Model file for the job. Use its own axes, mm. Face numbers are marked on the shaded views. A direction names the side the tool comes from. Give positions to 0.01 mm unless a question says otherwise; leave off trailing zeros. Order: outer loops, then holes, each group sorted by start corner. A loop starts at its lowest first (then second) coordinate and runs counter-clockwise, first axis right, second up. Notation, with made-up numbers: (34, 42) -> (71, 42) arc R35 ccw to (71, 81) -> close; hole circle Ø11 at (34.5, 63). An arc over 180 degrees is marked (long way). Answer in a Markdown table with one row per item. Add a question column.
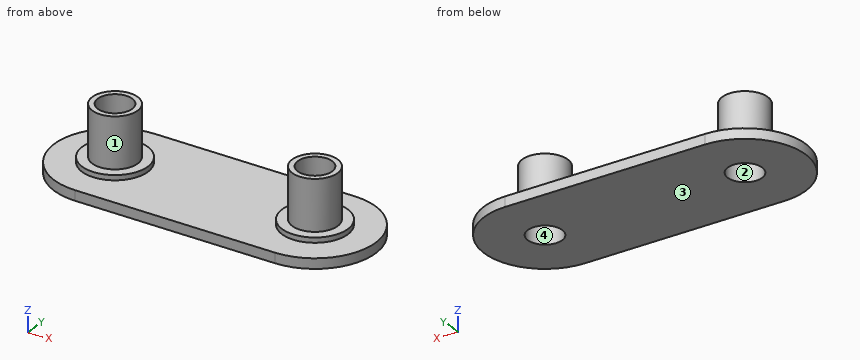
Autodesk Inventor part; units mm, degrees
ref_plane "YZ Plane" through (0, 0, 0) normal (1, 0, 0) x (0, 1, 0)
ref_plane "XZ Plane" through (0, 0, 0) normal (0, 1, 0) x (-1, 0, 0)
ref_plane "XY Plane" through (0, 0, 0) normal (0, 0, 1) x (1, 0, 0)
sketch "Sketch1" plane through (0, 0, 0) normal (0, 0, 1) x (1, 0, 0)
  line L0 (-10, 0) -> (10, 0) construction
  line L1 (-10, -6) -> (10, -6)
  line L2 (10, 6) -> (-10, 6)
  arc A0 (-10, 6) -> (-10, -6) centre (-10, 0) ccw
  arc A1 (10, -6) -> (10, 6) centre (10, 0) ccw
  circle A2 centre (-10, 0) radius 1.7
  circle A3 centre (10, 0) radius 1.7
  point P0 (0, 0)
  point P1 (0, 0)
  dimension "d0" = 20
  dimension "d1" = 6
  dimension "d2" = 3.4
extrude "Extrusion1" add sketch "Sketch1" along normal blind 1
sketch "Sketch2" plane through (0, 0, 1) normal (0, 0, 1) x (1, 0, 0)
  circle A0 centre (10, 0) radius 1.7
  circle A1 centre (10, 0) radius 2.25
  circle A2 centre (-10, 0) radius 1.7
  circle A3 centre (-10, 0) radius 2.25
  point P0 (0, 0)
  dimension "d5" = 4.5
  dimension "d6" = 4.5
extrude "Extrusion2" add sketch "Sketch2" along normal blind 5.5
sketch "Sketch3" plane through (0, 0, 1) normal (0, 0, 1) x (1, 0, 0)
  circle A0 centre (10, 0) radius 2.25
  circle A1 centre (-10, 0) radius 2.25
  circle A2 centre (10, 0) radius 2.25
  arc A3 (10, -6) -> (10, 6) centre (10, 0) ccw
  line L0 (10, 6) -> (-10, 6)
  arc A4 (-10, 6) -> (-10, -6) centre (-10, 0) ccw
  line L1 (-10, -6) -> (10, -6)
  circle A5 centre (10, 0) radius 3.25
  circle A6 centre (-10, 0) radius 3.25
  point P0 (0, 0)
  dimension "d9" = 6.5
extrude "Extrusion3" add sketch "Sketch3" along normal blind 0.5 contours A5 | A6
equation "\"d6\" = d5"
properties part number "Belt Retaining Guide"
Item 1: Saw through at C-C on x = 4.5. List the corners of the cut face in (y, z).
Item 2: Saw through at D-D on y = 4. List the corners of the cut face in (x, z), plus the area to 3 significant figures.
Item 3: Which spindle directions (+Z, -Z, +X, -X, +Y, -Y) get a long thin tool onto all of the face, cutting with end or side? Do the marked faces 1 and 2. Say none if no direction does.
Item 4: Saw through at A-A on y = 0. List the corners of the cut face in (x, z), plus the area to 3 significant figures.
Item 5: Two-plate mould, pull along X, no slides. Class the marked faces 3 and 4: pulls with the +X half, pulls with the -X half, needs draft (parallel to the pull), parting line crosses it, or undercut.
Item 6: Saw through at B-B on z = 5.25. List the corners of the cut face in (x, y).
Item 7: Wall check: line 1 (Y direction, x = 10, z = 3.5); line 2 (X direction, y = -1.5, z = 2.5); line 3 (Z direction, x = 6.5, y = 3). Give the ranges that are in metal, low to high.
Item 8: Pin check, flat tips, straight feed: pin 1 Ø6 at (x, y) = (-2.5, -0.5) entering from +Z; pin 2 Ø4.5 at (x, y) = (10, 0) entering from +Z; pin 3 Ø2 at (y, z) = (1, 5.5) entering from -X. Stop position of each tip, or through.
Evaluation:
| question | item | result |
|---|---|---|
| 1 | outline | (-6, 0) -> (6, 0) -> (6, 1) -> (-6, 1) -> close |
| 2 | outline | (-14.47, 0) -> (14.47, 0) -> (14.47, 1) -> (-14.47, 1) -> close |
| 2 | area | 28.9 mm2 |
| 3 | face 1 | +Z |
| 3 | face 2 | +Z, -Z |
| 4 | outline | (-16, 0) -> (-11.7, 0) -> (-11.7, 6.5) -> (-12.25, 6.5) -> (-12.25, 1.5) -> (-13.25, 1.5) -> (-13.25, 1) -> (-16, 1) -> close; (-8.3, 0) -> (8.3, 0) -> (8.3, 6.5) -> (7.75, 6.5) -> (7.75, 1.5) -> (6.75, 1.5) -> (6.75, 1) -> (-6.75, 1) -> (-6.75, 1.5) -> (-7.75, 1.5) -> (-7.75, 6.5) -> (-8.3, 6.5) -> close; (11.7, 0) -> (16, 0) -> (16, 1) -> (13.25, 1) -> (13.25, 1.5) -> (12.25, 1.5) -> (12.25, 6.5) -> (11.7, 6.5) -> close |
| 4 | area | 39.3 mm2 |
| 5 | face 3 | needs draft |
| 5 | face 4 | undercut |
| 6 | outline | circle Ø4.5 at (-10, 0); circle Ø4.5 at (10, 0); hole circle Ø3.4 at (-10, 0); hole circle Ø3.4 at (10, 0) |
| 7 | line 1 | y = -2.25 to -1.7, 1.7 to 2.25 |
| 7 | line 2 | x = -11.68 to -10.8, -9.2 to -8.32, 8.32 to 9.2, 10.8 to 11.68 |
| 7 | line 3 | z = 0 to 1 |
| 8 | pin 1 | stops at z = 1 |
| 8 | pin 2 | stops at z = 6.5 |
| 8 | pin 3 | stops at x = -12.25 |
